Geometry check sheet. Reference: the model listing, model coordinates, mm. Round coordinates to 2 decimals unless told otherwise and drop trailing zeros. Order: outer loops, then holes, each group sorted by start corner. A loop starts at its lowest first (then second) coordinate and runs counter-clockwise, first axis right, second up. Notation, with made-up numbers: (-35.5, -2.75) - (6.5, -2.75) arc R9 ccw to (6.5, 12.25) - close; hole circle Ø1 at (15, -39.5). An arc over 180 degrees is marked (long way). Use a Markdown table: item, result. Add a question column.
(1) Section check C-C on x = -10. Record the boundary of the cut face in (y, z) (3 decimals), then the cut area to 3 significant figures.
(2) Gauge pin test, flat ends, axial feed: P1, Ø1.5, axis at x = -60, y = -168.5, coming from the -Z side; P2, Ø1, axis at x = -51.5, z = 20.5, coming from the -Y side. Record the tip position at first contact, or that the pin passes through.
(3) Section check A-A on y = -169. Record the boundary of the cut face in (x, z).
(4) Thickness scan on line 1 along Z through (x, y) = (-14.5, -167.25); line 2 along Y through (x, z) = (-69, 21.5); line 3 along Z through (x, y) = (-61, -169.5). Record the ranges inside material, lowest first. Write a range as [from, to].
(5) Section check B-B on z = 22. Record the boundary of the cut face in (x, y), then the cut area to 3 significant figures.
```python
from build123d import *

# Parameters (mm, degrees)
BOSS_EXTRUDE2_OUTLINE_R = 3.175
BOSS_EXTRUDE2_DEPTH     = 146.812


# Read off the part's stored shape, not the designer's step: Boss-Extrude2
with BuildPart() as part:
    # Boss-Extrude2 outline → Boss-Extrude2 (new body)
    with BuildSketch(Plane(origin=(-98.013718438, 0, 0), x_dir=(0, 0, -1), z_dir=(1, 0, 0))):
        with Locations((-21.267819308, -167.583767489)):
            Circle(BOSS_EXTRUDE2_OUTLINE_R)
    extrude(amount=BOSS_EXTRUDE2_DEPTH)


solid = part.part
```
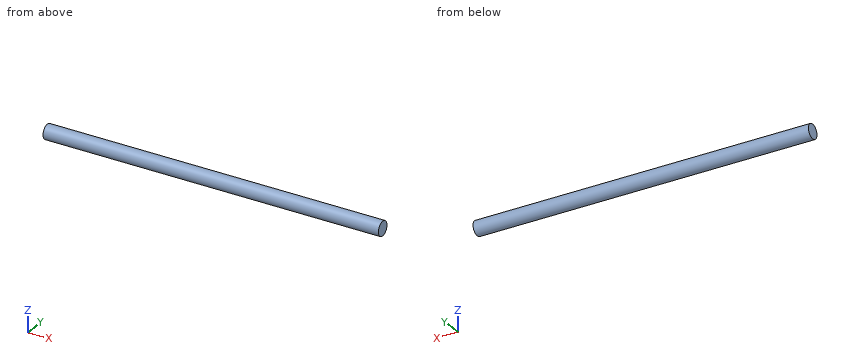
Check sheet entries:
| question | item | result |
|---|---|---|
| 1 | outline | circle Ø6.35 at (-167.584, 21.268) |
| 1 | area | 31.7 mm2 |
| 2 | P1 | stops at z = 18.1 |
| 2 | P2 | stops at y = -170.75 |
| 3 | outline | (-98.01, 18.43) - (48.8, 18.43) - (48.8, 24.11) - (-98.01, 24.11) - close |
| 4 | line 1 | z = [18.11, 24.43] |
| 4 | line 2 | y = [-170.75, -164.42] |
| 4 | line 3 | z = [18.74, 23.8] |
| 5 | outline | (-98.01, -170.67) - (48.8, -170.67) - (48.8, -164.49) - (-98.01, -164.49) - close |
| 5 | area | 907 mm2 |
